from build123d import *

# Parameters (mm, degrees)
SKETCH1_W               = 76.2
SKETCH1_H               = 34.925
BOSS_EXTRUDE1_DEPTH     = 2.54
SKETCH3_W               = 76.2
SKETCH3_H               = 3.81
BOSS_EXTRUDE3_DEPTH     = 5.08
SKETCH6_W               = 76.2
SKETCH6_H               = 2.54
BOSS_EXTRUDE4_DEPTH     = 1.27
SKETCH7_W               = 76.2
SKETCH7_H               = 2.54
BOSS_EXTRUDE5_DEPTH     = 1.27
FILL_START              = -15.231570796
FILL_PATTERN1_OUTLINE_R = 1.143
FILL_PATTERN1_DEPTH     = 29.845
SKETCH8_W               = 76.2
SKETCH8_H               = 2.54
BOSS_EXTRUDE6_DEPTH     = 1.27
SKETCH9_W               = 76.2
SKETCH9_H               = 2.54
BOSS_EXTRUDE7_DEPTH     = 1.27


# Read off the part's stored shape, not the designer's step: Fill Pattern1
with BuildPart() as part:
    # Sketch1 → Boss-Extrude1 (new body)
    with BuildSketch(Plane(origin=(0, 0, 0), x_dir=(1, 0, 0), z_dir=(0, 1, 0))):
        with Locations((1.784181416, 0.309070796)):
            Rectangle(SKETCH1_W, SKETCH1_H)
    extrude(amount=BOSS_EXTRUDE1_DEPTH)

    # Sketch3 → Boss-Extrude3 (add)
    with BuildSketch(Plane(origin=(0, 2.54, 0), x_dir=(1, 0, 0), z_dir=(0, 1, 0))):
        with Locations((1.784181416, 12.056570796)):
            Rectangle(SKETCH3_W, SKETCH3_H)
        with Locations((1.784181416, -11.438429204)):
            Rectangle(SKETCH3_W, SKETCH3_H)
    extrude(amount=BOSS_EXTRUDE3_DEPTH)

    # Sketch6 → Boss-Extrude4 (add)
    with BuildSketch(Plane.XY.offset(13.343429204)):
        with Locations((1.784181416, 6.35)):
            Rectangle(SKETCH6_W, SKETCH6_H)
    extrude(amount=BOSS_EXTRUDE4_DEPTH)

    # Sketch7 → Boss-Extrude5 (add)
    with BuildSketch(Plane(origin=(0, 0, -13.961570796), x_dir=(-1, 0, 0), z_dir=(0, 0, -1))):
        with Locations((-1.784181416, 6.35)):
            Rectangle(SKETCH7_W, SKETCH7_H)
    extrude(amount=BOSS_EXTRUDE5_DEPTH)

    # Fill Pattern1 outline → Fill Pattern1 (cut)
    with BuildSketch(Plane.XY.offset(FILL_START)):
        with Locations((1.784181416, 6.35)):
            Circle(FILL_PATTERN1_OUTLINE_R)
        with Locations((-10.915818584, 6.35)):
            Circle(FILL_PATTERN1_OUTLINE_R)
    extrude(amount=FILL_PATTERN1_DEPTH, mode=Mode.SUBTRACT)

    # Sketch8 → Boss-Extrude6 (add)
    with BuildSketch(Plane(origin=(0, 0, 9.533429204), x_dir=(-1, 0, 0), z_dir=(0, 0, -1))):
        with Locations((-1.784181416, 6.35)):
            Rectangle(SKETCH8_W, SKETCH8_H)
    extrude(amount=-BOSS_EXTRUDE6_DEPTH)

    # Sketch9 → Boss-Extrude7 (add)
    with BuildSketch(Plane.XY.offset(-10.151570796)):
        with Locations((1.784181416, 6.35)):
            Rectangle(SKETCH9_W, SKETCH9_H)
    extrude(amount=-BOSS_EXTRUDE7_DEPTH)


solid = part.part
Read the model definition and answer for the solid it produces. Units are mm, in the model's axes. A direction names the side the tool comes from. Round coordinates to 2 decimals unless told otherwise and drop trailing zeros. Loops run counter-clockwise (first coordinate to the right, second up) from the corner with the lowest first, then second, coordinate; pieces in that order, holes last.
Q1. Section B-B on x = -24 is taken. Write down the section's boundary in (y, z), and give its area (3 significant figures).
Q2. Section A-A on y = 6.35 is taken. Write down the section's boundary in (x, z).
Q3. Each of these flat-tipped pins is pushed along its axis until it touches: pin 1 (2 mm diameter, centred on x = -1.5, y = 6.5, fed in from +Z); pin 2 (2.5 mm diameter, centred on x = -11.5, y = 6, fed in from -Z); pin 3 (0.7 mm diameter, centred on x = 1.5, y = 6.5, fed in from +Z). Where does it stop, or does it pass through?
Q4. Determine the mould class of faces 4 (the face through (1, 4, 13.343)), 5 (the face through (-6, 6, -15.232)), 6 (the face through (1, 2.54, 0)) for opening direction Y: released by +Y, released by -Y, zero draft, split by the parting line, or undercut.
Q5. Consider probe 1 along X at (y, z) = (6.35, 13.65); probe 2 along X at (y, z) = (6.5, 13); probe 3 along Y at (x, z) = (2.5, -14). Determine where each line is inside the solid, lowest interval first.
Q6. Section C-C on z = 2 is taken. Write down the section's boundary in (x, y), and give its area (3 significant figures).
Q7. Which of the six approach directions +Z, -Z, +X, -X, +Y, -Y give full straight-line access (tool end or side, diameter ignored) to faces 1 (the face through (2.3, 5.08, -14.6)), 2 (the face through (1, 2.54, 15)), 3 (the face through (2, 6, -11.422))?
Output:
1. outline: (0, -17.77) - (2.54, -17.77) - (2.54, -13.96) - (5.08, -13.96) - (5.08, -15.23) - (7.62, -15.23) - (7.62, -10.15) - (2.54, -10.15) - (2.54, 9.53) - (7.62, 9.53) - (7.62, 14.61) - (5.08, 14.61) - (5.08, 13.34) - (2.54, 13.34) - (2.54, 17.15) - (0, 17.15) - close
1. area: 134 mm2
2. outline: (-36.32, -15.23) - (-12.06, -15.23) - (-12.06, -11.42) - (-9.77, -11.42) - (-9.77, -15.23) - (0.64, -15.23) - (0.64, -11.42) - (2.93, -11.42) - (2.93, -15.23) - (39.88, -15.23) - (39.88, -10.15) - (-36.32, -10.15) - close; (-36.32, 9.53) - (39.88, 9.53) - (39.88, 14.61) - (2.93, 14.61) - (2.93, 10.8) - (0.64, 10.8) - (0.64, 14.61) - (-9.77, 14.61) - (-9.77, 10.8) - (-12.06, 10.8) - (-12.06, 14.61) - (-36.32, 14.61) - close
3. pin 1: stops at z = 14.61
3. pin 2: stops at z = -15.23
3. pin 3: stops at z = 10.8
4. face 4: undercut
4. face 5: zero draft
4. face 6: released by +Y
5. probe 1: x = -36.32 to -12.06, -9.77 to 0.64, 2.93 to 39.88
5. probe 2: x = -36.32 to -12.05, -9.78 to 0.65, 2.92 to 39.88
5. probe 3: y = 0 to 2.54, 5.08 to 5.46, 7.24 to 7.62
6. outline: (-36.32, 0) - (39.88, 0) - (39.88, 2.54) - (-36.32, 2.54) - close
6. area: 194 mm2
7. face 1: -Z, +X, -X
7. face 2: +Z, +X, -X
7. face 3: -Z
